The listing builds one solid part. Answer for the finished solid, in the listing's coordinates (mm). A direction names the side the tool comes from. Give positions to 0.01 mm unless a question says otherwise; leave off trailing zeros. Order: outer loops, then holes, each group sorted by start corner. A loop starts at its lowest first (then second) coordinate and runs counter-clockwise, first axis right, second up.
```python
from build123d import *

# Parameters (mm, degrees)
SKETCH_3_R          = 3
CUT_EXTRUDE_1_DEPTH = 25.2


with BuildPart() as part:
    # 草圖2 → 旋轉1 (revolve)
    with BuildSketch(Plane(origin=(0, 0, 0), x_dir=(1, 0, 0), z_dir=(0, 1, 0))):
        Polygon((20, -0.5), (15.915, -1.85), (15.915, -22.35), (20, -23.7), (20, -24.2), (0, -24.2), (0, 0), (20, 0), align=None)
    revolve(axis=Axis((0, 0, 0), (0, 0, 1)))

    # 草圖3 → 除料-伸長1 (cut, through all)
    with BuildSketch(Plane.XY.offset(24.2)):
        Circle(SKETCH_3_R)
    extrude(amount=-CUT_EXTRUDE_1_DEPTH, mode=Mode.SUBTRACT)


solid = part.part
```
1) For a pull along Z with two mould halves and no side action, classify faces 3 (the conical face through (15.424, 4.857, 22.434)), 4 (the flat face through (4, 0, 24.2)), 5 (the cylindrical face through (-4.336, -19.524, 0.254)), 6 (the cylindrical face through (15.18, 4.78, 12.24)) as +Z half, -Z half, draft (parallel to the pull), parting line (faces both ways), or undercut.
Geometry says:
face 3: undercut
face 4: +Z half
face 5: draft
face 6: undercut
2) Find section C-C (z = 2.5). Write down the section's boundary in (x, y) (3 decimals), then the cut area to 3 significant figures.
Geometry says:
outline: circle Ø31.83 at (0, 0); hole circle Ø6 at (0, 0)
area: 767 mm2
3) Straight lines are drawn through the part: probe 1 along Y at (x, z) = (0, 18.25) (3 decimals); probe 2 along Z at (x, y) = (13, 15); probe 3 along X at (y, z) = (-2, 4). For each, find the intervals that lie inside material, in ascending order.
Geometry says:
probe 1: y = -15.915 to -3, 3 to 15.915
probe 2: z = 0 to 0.55, 23.65 to 24.2
probe 3: x = -15.79 to -2.24, 2.24 to 15.79
4) Find section A-A (y = 0). Write down the section's boundary in (x, z) (3 decimals).
Geometry says:
outline: (-20, 0) - (-3, 0) - (-3, 24.2) - (-20, 24.2) - (-20, 23.7) - (-15.915, 22.35) - (-15.915, 1.85) - (-20, 0.5) - close; (3, 0) - (20, 0) - (20, 0.5) - (15.915, 1.85) - (15.915, 22.35) - (20, 23.7) - (20, 24.2) - (3, 24.2) - close
5) Given P1, Ø4, axis at y = 13.5, z = 11.5, coming from the +X side; P2, Ø8, axis at y = -2.5, z = 10.5, coming from the +X side (3 decimals); P3, Ø5, axis at y = -15, z = 17.5, coming from the -X side; P4, Ø3.5, axis at x = 0, y = 0, coming from the +Z side, each flat-ended and moving along its own axis, determine where each tip first touches the part or whether it passes through.
Geometry says:
P1: stops at x = 11
P2: stops at x = 15.915
P3: stops at x = -9.85
P4: passes through
6) A tool of negligible diameter and unlimited length cuts with its end or side. For faces 1 (the cylindrical face through (-3, 0, 12)), 2 (the conical face through (-3.493, -15.73, 1.784)), from which of +Z, -Z, +X, -X, +Y, -Y can it reach the whole face along a straight path? Write none if from no direction.
Geometry says:
face 1: +Z, -Z
face 2: none
